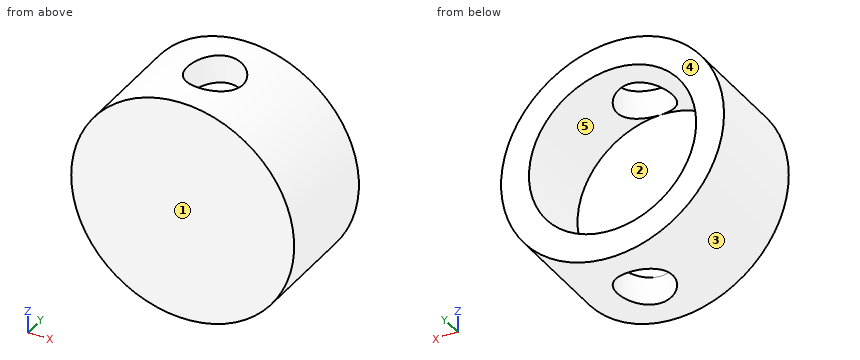
```python
from build123d import *

# Parameters (mm, degrees)
F0_W     = 25.4
F0_H     = 25.4
F1_DEPTH = 12.7
F2_R     = 3.175
F3_DEPTH = 25.4
F4_R     = 12.7
F5_DEPTH = 25.4
F6_R     = 9.525
F7_DEPTH = 9.525


with BuildPart() as f1:
    # F0 (on Front) → F1 (new body)
    with BuildSketch(Plane.XZ):
        Rectangle(F0_W, F0_H)
    extrude(amount=F1_DEPTH)

    # F2 (on face) → F3 (cut)
    with BuildSketch(Plane.XY.offset(12.7)):
        with Locations((0, -6.35)):
            Circle(F2_R)
    extrude(amount=-F3_DEPTH, mode=Mode.SUBTRACT)

    # F4 (on face) → F5 (intersect)
    with BuildSketch(Plane(origin=(0, 0, 0), x_dir=(-1, 0, 0), z_dir=(0, 1, 0))):
        Circle(F4_R)
    extrude(amount=-F5_DEPTH, mode=Mode.INTERSECT)

    # F6 (on face) → F7 (cut)
    with BuildSketch(Plane(origin=(0, 0, 0), x_dir=(-1, 0, 0), z_dir=(0, 1, 0))):
        Circle(F6_R)
    extrude(amount=-F7_DEPTH, mode=Mode.SUBTRACT)


solid = f1.part
```
Check sheet for the modelled part. Datum: model origin and axes. Units: mm. Face numbers are marked on the shaded views. A direction names the side the tool comes from. Coordinates: 2 decimals unless noted, no trailing zeros. Write each loop counter-clockwise with the first axis right and the second up, starting at its lowest first coordinate (ties: lowest second). Pieces come first, ordered by that corner, then holes. Notation, with made-up numbers: (77.25, -37) - (120.25, -37) arc R26 cw to (120.25, -13) - close; hole circle Ø5 at (-22.5, 3). An arc over 180 degrees is marked (long way). One line per question, with ' | ' between items.
Item 1: Sectioned sample at A-A on x = 1. Record the boundary of the cut face in (y, z) (3 decimals).
Determined:
outline: (-12.7, -12.661) - (-9.363, -12.661) - (-9.363, -9.472) - (-9.525, -9.472) - (-9.525, 9.472) - (-9.363, 9.472) - (-9.363, 12.661) - (-12.7, 12.661) - close; (-3.337, -12.661) - (0, -12.661) - (0, -9.472) - (-3.337, -9.472) - close; (-3.337, 9.472) - (0, 9.472) - (0, 12.661) - (-3.337, 12.661) - close
Item 2: Mould release check, pull along Z, two halves, no side actions. Record for the marked faces 1, 2 and 3: pulls with the +Z half, pulls with the -Z half, needs draft (parallel to the pull), parting line crosses it, or undercut.
Determined:
face 1: needs draft | face 2: undercut | face 3: parting line crosses it
Item 3: Sectioned sample at D-D on y = -1.5. Record the boundary of the cut face in (x, z) (3 decimals).
Determined:
outline: circle Ø25.4 at (0, 0); hole circle Ø19.05 at (0, 0)
Item 4: Thickness scan on line 1 (Z direction, x = 0, y = -2.5) (3 decimals); line 2 (Y direction, x = 0, z = 11.1) (3 decimals). Record the ranges inside material, lowest first. Write a range as [from, to].
Determined:
line 1: z = [-12.7, -9.525], [9.525, 12.7] | line 2: y = [-12.7, -9.525], [-3.175, 0]
Item 5: Gauge pin test, flat ends, axial feed: P1, Ø5, axis at x = 0, y = -6.35, coming from the -Z side; P2, Ø1.5, axis at y = -3.5, z = 2.5, coming from the +X side; P3, Ø4, axis at x = 4, y = -3, coming from the -Z side; P4, Ø4, axis at y = -2, z = -7.5, coming from the +X side. Record the tip position at first contact, or that the pin passes through.
Determined:
P1: passes through | P2: stops at x = 12.58 | P3: stops at z = -12.54 | P4: stops at x = 11.45
Item 6: Sectioned sample at C-C on y = -6. Record the boundary of the cut face in (x, z) (3 decimals), plus the area to 3 significant figures.
Determined:
outline: (-3.156, -12.302) - (-3.156, -8.987) arc R9.525 cw to (-3.156, 8.987) - (-3.156, 12.302) arc R12.7 ccw to start; (3.156, -12.302) arc R12.7 ccw to (3.156, 12.302) - (3.156, 8.987) arc R9.525 cw to (3.156, -8.987) - close | area: 181 mm2
Item 7: Access from +Z, -Z, +X, -X, +Y, -Y to the whole of each face (thin tool, end or side, straight path). Record for the marked faces 4 and 5.
Determined:
face 4: +Z, -Z, +X, -X, +Y | face 5: +Y
Item 8: Sectioned sample at B-B on z = 0. Record the boundary of the cut face in (x, y) (3 decimals), plus the area to 3 significant figures.
Determined:
outline: (-12.7, -12.7) - (12.7, -12.7) - (12.7, 0) - (9.525, 0) - (9.525, -9.525) - (-9.525, -9.525) - (-9.525, 0) - (-12.7, 0) - close | area: 141 mm2
